```python
from build123d import *

# Parameters (mm, degrees)
F1_DEPTH = 2
F3_DEPTH = 1


with BuildPart() as f1:
    # F0 (on Top) → F1 (new body)
    with BuildSketch(Plane.XY):
        with BuildLine():
            ThreePointArc((-17.746939, -22.999996), (-17.161152, -24.41421), (-15.746939, -24.999996))
            Line((-15.746939, -24.999996), (15.253061, -24.999996))
            ThreePointArc((15.253061, -24.999996), (16.667275, -24.41421), (17.253061, -22.999996))
            Line((17.253061, -22.999996), (17.253061, 23.000004))
            ThreePointArc((17.253061, 23.000004), (16.667275, 24.414217), (15.253061, 25.000004))
            Line((15.253061, 25.000004), (-15.746939, 25.000004))
            ThreePointArc((-15.746939, 25.000004), (-17.161152, 24.414217), (-17.746939, 23.000004))
            Line((-17.746939, 23.000004), (-17.746939, -22.999996))
        make_face()
    extrude(amount=F1_DEPTH)

    # F2 (on face) → F3 (join)
    with BuildSketch(Plane.XY.offset(2)):
        with BuildLine():
            Line((20.253061, -22.999996), (20.253061, 23.000004))
            ThreePointArc((20.253061, 23.000004), (18.788595, 26.535538), (15.253061, 28.000004))
            Line((15.253061, 28.000004), (-15.746939, 28.000004))
            ThreePointArc((-15.746939, 28.000004), (-19.282472, 26.535538), (-20.746939, 23.000004))
            Line((-20.746939, 23.000004), (-20.746939, -22.999996))
            ThreePointArc((-20.746939, -22.999996), (-19.282472, -26.53553), (-15.746939, -27.999996))
            Line((-15.746939, -27.999996), (15.253061, -27.999996))
            ThreePointArc((15.253061, -27.999996), (18.788595, -26.53553), (20.253061, -22.999996))
        make_face()
    extrude(amount=-F3_DEPTH)


solid = f1.part
```
The listing builds one solid part. Answer for the finished solid, in the listing's coordinates (mm). A direction names the side the tool comes from. Round coordinates to 2 decimals unless told otherwise and drop trailing zeros. Loops run counter-clockwise (first coordinate to the right, second up) from the corner with the lowest first, then second, coordinate; pieces in that order, holes last. Notation, with made-up numbers: (28.25, -14.75) - (33.25, -14.75) arc R20 ccw to (33.25, 22.25) - close; hole circle Ø8 at (64, 70.25). An arc over 180 degrees is marked (long way). Return JSON: item names as keys, results as strings. Group by question number.
1. Each of these flat-tipped pins is pushed along its axis until it touches: P1, Ø0.5, axis at x = -5.5, z = 0.5, coming from the +Y side; P2, Ø0.8, axis at y = 6, z = 0.5, coming from the -X side. Where does it stop, or does it pass through?
2. Which of the six approach directions +Z, -Z, +X, -X, +Y, -Y give full straight-line access (tool end or side, diameter ignored) to faces 1 (the cylindrical face through (-17.146, 24.43, 0.493)), 2 (the cylindrical face through (16.68, 24.4, 0.49)), 3 (the flat face through (-19, 2, 1)), 4 (the cylindrical face through (16.65, -24.43, 0.49))?
3. The part is cut by section B-B on y = -12. Determine the outline of the cut face in (x, z), then the cut area to 3 significant figures.
4. Consider probe 1 along Y at (x, z) = (-5.5, 0.4); probe 2 along Z at (x, y) = (18.5, -5); probe 3 along X at (y, z) = (-7, 0.55). Determine where each line is inside the solid, lowest interval first.
5. The part is cut by section A-A on x = 14. Determine the outline of the cut face in (y, z), then the cut area to 3 significant figures.
Resolved:
{
 "1": {"P1": "stops at y = 25", "P2": "stops at x = -17.75"},
 "2": {"face 1": "-Z, -X, +Y", "face 2": "-Z, +X, +Y", "face 3": "-Z", "face 4": "-Z, +X, -Y"},
 "3": {"outline": "(-20.75, 1) - (-17.75, 1) - (-17.75, 0) - (17.25, 0) - (17.25, 1) - (20.25, 1) - (20.25, 2) - (-20.75, 2) - close", "area": "76.0 mm²"},
 "4": {"probe 1": "y = -25 to 25", "probe 2": "z = 1 to 2", "probe 3": "x = -17.75 to 17.25"},
 "5": {"outline": "(-28, 1) - (-25, 1) - (-25, 0) - (25, 0) - (25, 1) - (28, 1) - (28, 2) - (-28, 2) - close", "area": "106 mm²"}
}
